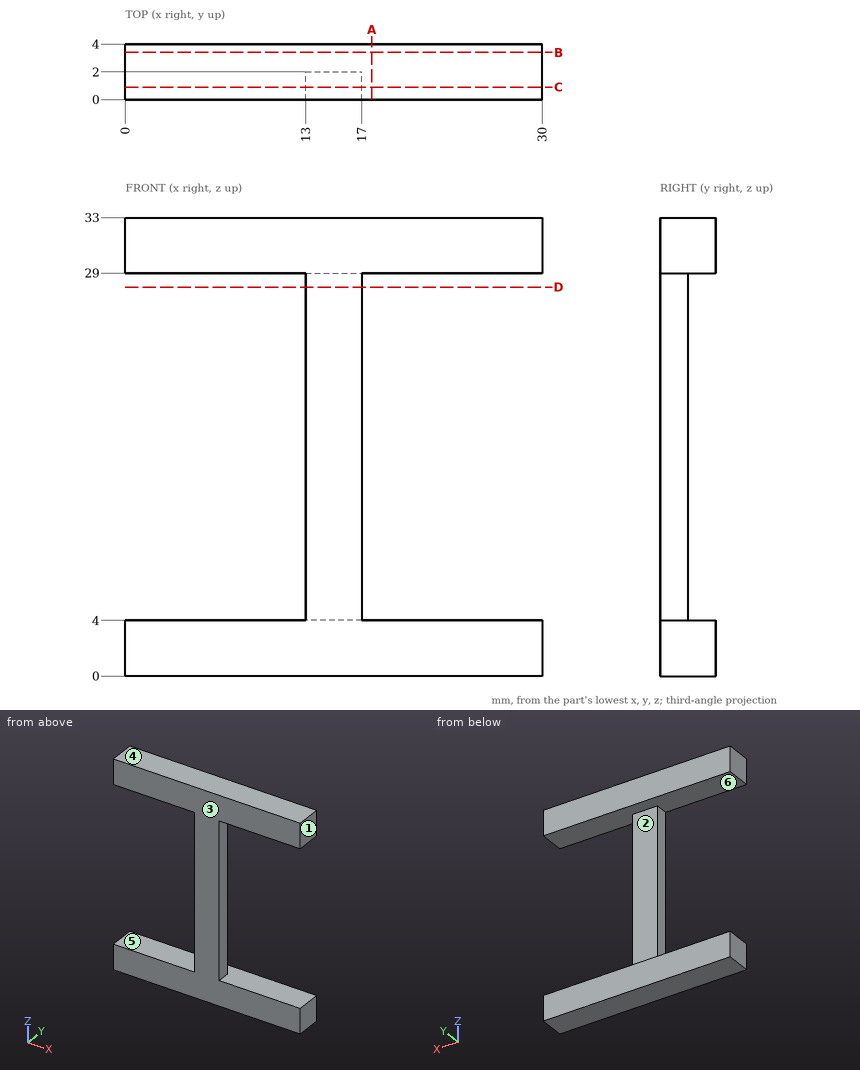
Geometry check sheet. Reference: drawing and pictorial views, mm from the part's lowest x, y, z. A direction names the side the tool comes from. Give positions to 0.01 mm unless a question says otherwise; leave off trailing zeros. Write each loop counter-clockwise with the first axis right and the second up, starting at its lowest first coordinate (ties: lowest second). Pieces come first, ordered by that corner, then holes. Notation, with made-up numbers: (78.5, -33.75) - (101.5, -33.75) arc R20 ccw to (101.5, -12.75) - close; hole circle Ø6 at (-2, 50.5). An arc over 180 degrees is marked (long way). Use a Markdown table: item, result.
Q1. Section check D-D, the plane z = 28. Enter the section's corners in (x, y), then the cut area to 3 significant figures.
Computed:
| item | result |
|---|---|
| outline | (13, 0) - (17, 0) - (17, 2) - (13, 2) - close |
| area | 8.00 mm² |
Q2. Section check A-A, the plane x = 17.75. Enter the section's corners in (y, z).
Computed:
| item | result |
|---|---|
| outline | (0, 0) - (4, 0) - (4, 4) - (0, 4) - close; (0, 29) - (4, 29) - (4, 33) - (0, 33) - close |
Q3. Thickness scan on L1, parallel to Z at x = 28, y = 2.9; L2, parallel to X at y = 1.8, z = 27. Record the ranges inside material, lowest first. Write a range as [from, to].
Computed:
| item | result |
|---|---|
| L1 | z = [0, 4], [29, 33] |
| L2 | x = [13, 17] |
Q4. Draft check along Z on the marked faces 3, 4, 5 and 6. Enter one of: pulls with the +Z half, pulls with the -Z half, needs draft (parallel to the pull), parting line crosses it, or undercut.
Computed:
| item | result |
|---|---|
| face 3 | needs draft |
| face 4 | pulls with the +Z half |
| face 5 | undercut |
| face 6 | undercut |
Q5. Section check C-C, the plane y = 0.9. Enter the section's corners in (x, z), then the cut area to 3 significant figures.
Computed:
| item | result |
|---|---|
| outline | (0, 0) - (30, 0) - (30, 4) - (17, 4) - (17, 29) - (30, 29) - (30, 33) - (0, 33) - (0, 29) - (13, 29) - (13, 4) - (0, 4) - close |
| area | 340 mm² |
Q6. Go/stop test with flat-tipped pins: P1, Ø0.6, axis at y = 1, z = 13, coming from the -X side; P2, Ø1.5, axis at x = 4.5, y = 1, coming from the -Z side; P3, Ø2, axis at y = 1, z = 16, coming from the +X side; P4, Ø2, axis at x = 15.5, z = 22.5, coming from the +Y side. Record where each tip stops, or that it passes through.
Computed:
| item | result |
|---|---|
| P1 | stops at x = 13 |
| P2 | stops at z = 0 |
| P3 | stops at x = 17 |
| P4 | stops at y = 2 |
Q7. Section check B-B, the plane y = 3.4. Enter the section's corners in (x, z).
Computed:
| item | result |
|---|---|
| outline | (0, 0) - (30, 0) - (30, 4) - (0, 4) - close; (0, 29) - (30, 29) - (30, 33) - (0, 33) - close |
Q8. Set-up check for the marked faces 1 and 2: record each of +Z, -Z, +X, -X, +Y, -Y from which the full face is reachable in a straight line by a thin tool's end or side.
Computed:
| item | result |
|---|---|
| face 1 | +Z, -Z, +X, +Y, -Y |
| face 2 | +X, -X, +Y |
